For this review, use the dimensioned drawing (mm, ordinates from the lowest corner) and the shaded views. A direction names the side the tool comes from. Coordinates: 2 decimals unless noted, no trailing zeros. Loops run counter-clockwise (first coordinate to the right, second up) from the corner with the lowest first, then second, coordinate; pieces in that order, holes last.
1. Take a section at B-B, the plane z = 2.84. State the section outline as (x, y) points.
2. Clearance check with flat-ended pins moving along their axes: P1, Ø2, axis at x = 3.5, y = 5, coming from the -Z side; P2, Ø3, axis at x = 1.5, z = 1, coming from the -Y side. State where each tip first meets the part, or that it passes through.
3. Mouldability with a two-part tool opening along X and no side actions: class the marked faces 1, 2, 3 and 4 as pulls with the +X half, pulls with the -X half, needs draft (parallel to the pull), parting line crosses it, or undercut.
4. Take a section at C-C, the plane y = 4.75. State the section outline as (x, z) points.
5. To check wall thickness, follow probe 1 along Y at (x, z) = (0.9, 2.85); probe 2 along Y at (x, z) = (3.45, 2.75); probe 3 along Z at (x, y) = (3.6, 6) (1 decimal). State the ranges of each line that lie inside material, in increasing order.
6. Machinability: for the marked faces 5, 6 and 7, which of the approach directions +Z, -Z, +X, -X, +Y, -Y give a long, thin tool a straight path to every point of the face, cutting with its end or side? Answer none if there is none.
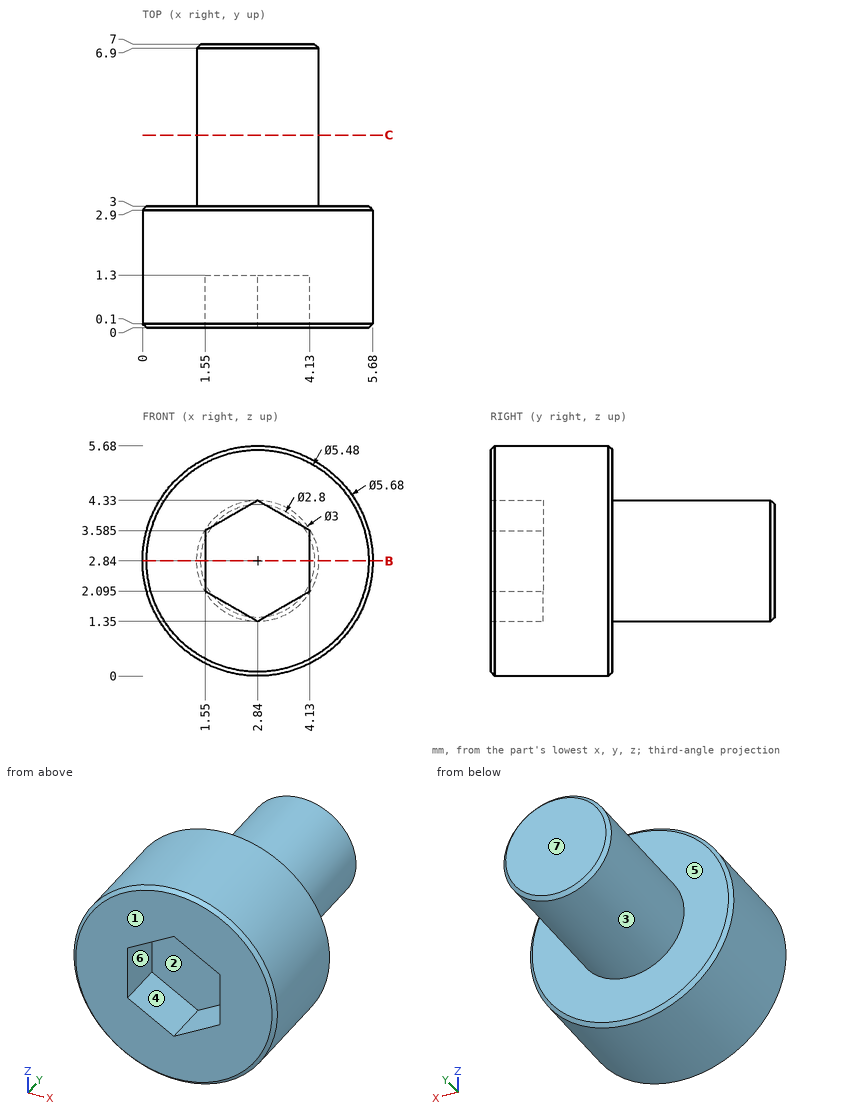
Results list:
1. outline: (0, 0.1) - (0.1, 0) - (1.55, 0) - (1.55, 1.3) - (4.13, 1.3) - (4.13, 0) - (5.58, 0) - (5.68, 0.1) - (5.68, 2.9) - (5.58, 3) - (4.34, 3) - (4.34, 6.9) - (4.24, 7) - (1.44, 7) - (1.34, 6.9) - (1.34, 3) - (0.1, 3) - (0, 2.9) - close
2. P1: stops at z = 1.34
2. P2: stops at y = 0
3. face 1: needs draft
3. face 2: undercut
3. face 3: parting line crosses it
3. face 4: undercut
4. outline: circle Ø3 at (2.84, 2.84)
5. probe 1: y = 0 to 3
5. probe 2: y = 1.3 to 7
5. probe 3: z = 1.5 to 4.1
6. face 5: +Y
6. face 6: -Y
6. face 7: +Z, -Z, +X, -X, +Y
